Build history of the part. All positions in model axes, mm. A direction names the side the tool comes from. Give positions to 0.01 mm unless a question says otherwise; leave off trailing zeros. Order: outer loops, then holes, each group sorted by start corner. A loop starts at its lowest first (then second) coordinate and runs counter-clockwise, first axis right, second up. Notation, with made-up numbers: M 49,-12 L 81,-12 A13 cw 81,-6 Z; hole C -3,45 d8. An arc over 180 degrees is marked long. One line per item, written item: value.
from build123d import *

# Parameters (mm, degrees)
SKETCH1_W           = 300
SKETCH1_H           = 100
BOSS_EXTRUDE1_DEPTH = 10
SKETCH2_W           = 20
SKETCH2_H           = 100
BOSS_EXTRUDE2_DEPTH = 90
SKETCH3_W           = 19.9
SKETCH3_H           = 40.9
SKETCH3_R           = 0.75
CUT_EXTRUDE1_DEPTH  = 321.156211872
SKETCH4_W           = 100
SKETCH4_H           = 10
BOSS_EXTRUDE4_DEPTH = 60
SKETCH6_W           = 200
SKETCH6_H           = 10
BOSS_EXTRUDE5_DEPTH = 10
FILLET1_R           = 2
SKETCH8_W           = 20
SKETCH8_H           = 100
BOSS_EXTRUDE7_DEPTH = 50
BOSS_EXTRUDE9_DEPTH = 300
SKETCH12_W          = 260
SKETCH12_H          = 100
CUT_EXTRUDE4_DEPTH  = 20
SKETCH13_R          = 1.5
CUT_EXTRUDE5_DEPTH  = 207.639783198
SKETCH14_R          = 7.15
CUT_EXTRUDE7_DEPTH  = 335.813380856
SKETCH15_R          = 1.5
CUT_EXTRUDE8_DEPTH  = 212.187120819


with BuildPart() as part:
    # Sketch1 → Boss-Extrude1 (new body)
    with BuildSketch(Plane.XY):
        Rectangle(SKETCH1_W, SKETCH1_H)
    extrude(amount=BOSS_EXTRUDE1_DEPTH)

    # Sketch2 → Boss-Extrude2 (add)
    with BuildSketch(Plane.XY.offset(10)):
        with Locations((-140, 0)):
            Rectangle(SKETCH2_W, SKETCH2_H)
        with Locations((140, 0)):
            Rectangle(SKETCH2_W, SKETCH2_H)
    extrude(amount=BOSS_EXTRUDE2_DEPTH)

    # Sketch3 → Cut-Extrude1 (cut, through all)
    with BuildSketch(Plane.ZY.offset(150)):
        with Locations((50, 0)):
            Rectangle(SKETCH3_W, SKETCH3_H)
        with Locations((45.025, 21.95)):
            Circle(SKETCH3_R)
        with Locations((54.975, 21.95)):
            Circle(SKETCH3_R)
        with Locations((45.025, -21.95)):
            Circle(SKETCH3_R)
        with Locations((54.975, -21.95)):
            Circle(SKETCH3_R)
    extrude(amount=-CUT_EXTRUDE1_DEPTH, mode=Mode.SUBTRACT)

    # Sketch4 → Boss-Extrude4 (add)
    with BuildSketch(Plane.XZ.offset(50)):
        with Locations((0, 5)):
            Rectangle(SKETCH4_W, SKETCH4_H)
    extrude(amount=BOSS_EXTRUDE4_DEPTH)

    # Sketch6 → Boss-Extrude5 (add)
    with BuildSketch(Plane.XZ.offset(110)):
        with Locations((0, 5)):
            Rectangle(SKETCH6_W, SKETCH6_H)
    extrude(amount=-BOSS_EXTRUDE5_DEPTH)

    # Fillet1
    fillet1_edges = [part.edges().sort_by_distance(p)[0] for p in [
        (-100, -110, 5),
        (100, -100, 5),
        (-100, -100, 5),
        (100, -110, 5),
    ]]
    fillet(fillet1_edges, radius=FILLET1_R)

    # Sketch8 → Boss-Extrude7 (add)
    with BuildSketch(Plane(origin=(0, 50, 0), x_dir=(1, 0, 0), z_dir=(0, 1, 0))):
        with Locations((-140, -50)):
            Rectangle(SKETCH8_W, SKETCH8_H)
        with Locations((140, -50)):
            Rectangle(SKETCH8_W, SKETCH8_H)
    extrude(amount=BOSS_EXTRUDE7_DEPTH)

    # Sketch9 → Boss-Extrude9 (add, through all)
    with BuildSketch(Plane.ZY.offset(150)):
        with BuildLine():
            Line((0, 108), (0, 102.5))
            Line((0, 102.5), (48.5, 102.5))
            ThreePointArc((48.5, 102.5), (50, 104), (51.5, 102.5))
            Line((51.5, 102.5), (100, 102.5))
            Line((100, 102.5), (100, 108))
            Line((100, 108), (0, 108))
        make_face()
        with BuildLine():
            Line((0, 102.5), (0, 100))
            Line((0, 100), (100, 100))
            Line((100, 100), (100, 102.5))
            Line((100, 102.5), (51.5, 102.5))
            ThreePointArc((51.5, 102.5), (50, 101), (48.5, 102.5))
            Line((48.5, 102.5), (0, 102.5))
        make_face()
    extrude(amount=-BOSS_EXTRUDE9_DEPTH)

    # Sketch12 → Cut-Extrude4 (cut)
    with BuildSketch(Plane.XZ.offset(-100)):
        with Locations((0, 50)):
            Rectangle(SKETCH12_W, SKETCH12_H)
    extrude(amount=-CUT_EXTRUDE4_DEPTH, mode=Mode.SUBTRACT)

    # Sketch13 → Cut-Extrude5 (cut, through all)
    with BuildSketch(Plane.XY.offset(10)):
        with Locations((12.5, -35)):
            Circle(SKETCH13_R)
        with Locations((12.5, -40)):
            Circle(SKETCH13_R)
        with Locations((12.5, -45)):
            Circle(SKETCH13_R)
        with Locations((-12.5, -35)):
            Circle(SKETCH13_R)
        with Locations((-12.5, -40)):
            Circle(SKETCH13_R)
        with Locations((-12.5, -45)):
            Circle(SKETCH13_R)
    extrude(amount=-CUT_EXTRUDE5_DEPTH, mode=Mode.SUBTRACT)

    # Sketch14 → Cut-Extrude7 (cut, through all)
    with BuildSketch(Plane(origin=(150, 0, 0), x_dir=(0, 0, -1), z_dir=(1, 0, 0))):
        with Locations(Location((-50.372507489, 99.940398802, 0), (0, 0, 90))):
            Circle(SKETCH14_R)
    extrude(amount=-CUT_EXTRUDE7_DEPTH, mode=Mode.SUBTRACT)

    # Sketch15 → Cut-Extrude8 (cut, through all)
    with BuildSketch(Plane(origin=(0, 0, 0), x_dir=(-1, 0, 0), z_dir=(0, 0, -1))):
        with Locations((-17.5, 45.680401999)):
            Circle(SKETCH15_R)
        with Locations((17.5, 45.680401999)):
            Circle(SKETCH15_R)
        with Locations((-17.5, 30.680401999)):
            Circle(SKETCH15_R)
        with Locations((17.5, 30.786051179)):
            Circle(SKETCH15_R)
    extrude(amount=-CUT_EXTRUDE8_DEPTH, mode=Mode.SUBTRACT)


solid = part.part
1) Tool access for faces 4 (the face through (140, 20.45, 50)), 5 (the face through (-74, -100, 5)), 6 (the face through (133, -50, 35)), 7 (the face through (-2, 50, 5)), 8 (the face through (-2, -13, 10)): list every direction of +Z, -Z, +X, -X, +Y, -Y with a clear straight run to the whole face (end or side of a thin tool).
Check values:
face 4: +X, -X
face 5: +Z, -Z, -X
face 6: +Z, -Z, +X
face 7: +Z, -Z, +Y
face 8: +Z, +Y, -Y
2) Saw through at B-B, the plane y = 74. Write the cut outline in (x, z).
Check values:
outline: M -150,0 L -130,0 L -130,100 L -150,100 Z; M 130,0 L 150,0 L 150,100 L 130,100 Z
3) Drill centre lines: probe 1 along Y at (x, z) = (12.5, 5.75); probe 2 along X at (y, z) = (62, 21); probe 3 along Y at (x, z) = (17.5, 2.5). Where is each one in solid material? Low to high. Write a range as from..to.
Check values:
probe 1: -110..-46.5, -43.5..-41.5, -38.5..-36.5, -33.5..50
probe 2: -150..-130, 130..150
probe 3: -110..29.18, 32.18..44.18, 47.18..50
4) Saw through at C-C, the plane y = 11. Write the cut outline in (x, z).
Check values:
outline: M -150,0 L 150,0 L 150,40.05 L 130,40.05 L 130,10 L -130,10 L -130,40.05 L -150,40.05 Z; M -150,59.95 L -130,59.95 L -130,100 L -150,100 Z; M 130,59.95 L 150,59.95 L 150,100 L 130,100 Z
5) Saw through at A-A, the plane z = 72.5. Write the cut outline in (x, y).
Check values:
outline: M -150,-50 L -130,-50 L -130,108 L -150,108 Z; M 130,-50 L 150,-50 L 150,108 L 130,108 Z
6) Mould opens along Y. For faces 1 (the face through (-140, 108, 51)), 2 (the face through (140, -20.45, 50)), 3 (the face through (130, 28, 49)) say: released by +Y, released by -Y, zero draft, split by the parting line, or undercut.
Check values:
face 1: released by +Y
face 2: undercut
face 3: zero draft
7) Pin check, flat tips, straight feed: pin 1 (6 mm diameter, centred on x = 142, z = 54, fed in from -Y); pin 2 (5 mm diameter, centred on y = -75, z = 7, fed in from -X); pin 3 (3 mm diameter, centred on y = -68, z = 4.5, fed in from +X). Stop position of each tip, or through.
Check values:
pin 1: y = -50
pin 2: x = -50
pin 3: x = 50
8) Saw through at D-D, the plane y = 37.5. Write the cut outline in (x, z).
Check values:
outline: M -150,0 L 150,0 L 150,100 L 130,100 L 130,10 L -130,10 L -130,100 L -150,100 Z
